Can you work these out from the model? Positions are in its coordinate system, mm. A direction names the side the tool comes from. Give positions to 0.01 mm unless a question says otherwise; leave off trailing zeros. Order: outer loops, then holes, each group sorted by start corner. A loop starts at its lowest first (then second) coordinate and runs counter-clockwise, first axis right, second up. Notation, with made-up numbers: (50, 11) - (105, 11) arc R19 cw to (105, 29) - close; hole circle Ø4 at (25, 64.25). An arc over 180 degrees is marked (long way). Answer as CSV lines item,"result".
```python
from build123d import *

# Parameters (mm, degrees)
SKETCH_1_R               = 2.5
EXTRUDE_1_DEPTH          = 4
EXTRUDE_2_DEPTH          = 15
SKETCH_3_W               = 28
SKETCH_3_H               = 4
CUT_EXTRUDE_1_DEPTH      = 8
CUT_EXTRUDE_2_DEPTH      = 60.149678768
CUT_EXTRUDE_2_DEPTH_BACK = 60.149678768


with BuildPart() as part:
    # 草图1 → 凸台-拉伸1 (new body)
    with BuildSketch(Plane(origin=(0, 0, 0), x_dir=(1, 0, 0), z_dir=(0, 1, 0))):
        with BuildLine():
            Line((-27.928932188, -4.947284101), (27.928932188, -4.947284101))
            ThreePointArc((27.928932188, -4.947284101), (32.548329851, -8.03386694), (31.464466094, -13.482818007))
            Line((31.464466094, -13.482818007), (3.535533906, -41.411750195))
            ThreePointArc((3.535533906, -41.411750195), (0, -42.87621629), (-3.535533906, -41.411750195))
            Line((-3.535533906, -41.411750195), (-31.464466094, -13.482818007))
            ThreePointArc((-31.464466094, -13.482818007), (-32.548329851, -8.03386694), (-27.928932188, -4.947284101))
        make_face()
        with Locations(Location((-25, -9.947284101, 0), (0, 0, 270))):
            Circle(SKETCH_1_R, mode=Mode.SUBTRACT)
        with Locations(Location((25, -9.947284101, 0), (0, 0, 270))):
            Circle(SKETCH_1_R, mode=Mode.SUBTRACT)
        with Locations(Location((0, -34.947284101, 0), (0, 0, 270))):
            Circle(SKETCH_1_R, mode=Mode.SUBTRACT)
    extrude(amount=EXTRUDE_1_DEPTH)

    # 草图2 → 凸台-拉伸2 (add)
    with BuildSketch(Plane(origin=(0, 0, 4.947284101), x_dir=(-1, 0, 0), z_dir=(0, 0, -1))):
        Polygon((-20, 4), (-8.452994616, 24), (8.452994616, 24), (20, 4), align=None)
    extrude(amount=-EXTRUDE_2_DEPTH)

    # 草图3 → 切除-拉伸1 (cut)
    with BuildSketch(Plane(origin=(0, 0, 4.947284101), x_dir=(-1, 0, 0), z_dir=(0, 0, -1))):
        with Locations((0, 2)):
            Rectangle(SKETCH_3_W, SKETCH_3_H)
    extrude(amount=-CUT_EXTRUDE_1_DEPTH, mode=Mode.SUBTRACT)

    # 草图4 → 切除-拉伸2 (cut, two sides: drawn at the far end of the back side and taken through both)
    with BuildSketch(Plane(origin=(0, 0, 0), x_dir=(0, 0, -1), z_dir=(1, 0, 0)).offset(-CUT_EXTRUDE_2_DEPTH_BACK)):
        Polygon((-19.947284101, 24), (-7.947284101, 24), (-19.947284101, 4), align=None)
    extrude(amount=CUT_EXTRUDE_2_DEPTH + CUT_EXTRUDE_2_DEPTH_BACK, mode=Mode.SUBTRACT)


solid = part.part
```
1) I'm going to push flat-ended pins straight in: P1, Ø8, axis at x = 11, y = 20, coming from the -Z side; P2, Ø1.2, axis at x = -2.5, y = 3, coming from the -Z side; P3, Ø3, axis at y = 2, z = 7.5, coming from the +X side; P4, Ø4, axis at x = 13.5, y = 3, coming from the +Z side. Where does each tip first touch, or does it pass through?
Answer block:
P1,"z = 4.95"
P2,"z = 12.95"
P3,"x = 32.84"
P4,"z = 33.45"
2) I need wall thicknesses on line 1 along Y through (x, z) = (14, 21.5); line 2 along X through (y, z) = (12.5, 7); line 3 along Y through (x, z) = (-6, 19). Which ranges of each line are inside material? Lowest first, please. Write a range as [from, to].
Answer block:
line 1,"[0, 4]"
line 2,"[-15.09, 15.09]"
line 3,"[0, 5.58]"
3) I want a section at B-B on y = 2.5. Write out the boundary of the cut face in (x, z), plus the area to 3 significant figures.
Answer block:
outline,"(-31.46, 13.48) arc R5 ccw to (-27.93, 4.95) - (-14, 4.95) - (-14, 12.95) - (14, 12.95) - (14, 4.95) - (27.93, 4.95) arc R5 ccw to (31.46, 13.48) - (3.54, 41.41) arc R5 ccw to (-3.54, 41.41) - close; hole circle Ø5 at (-25, 9.95); hole circle Ø5 at (0, 34.95); hole circle Ø5 at (25, 9.95)"
area,"1,250 mm2"
4) I want a section at D-D on x = 7. Write out the boundary of the cut face in (y, z).
Answer block:
outline,"(0, 12.95) - (4, 12.95) - (4, 4.95) - (24, 4.95) - (24, 7.95) - (4, 19.95) - (4, 37.95) - (0, 37.95) - close"
5) If we mould it in two halves opening along X, with no side actions, what happens to faces 4 (the flat face through (0, 2, 12.947)), 5 (the flat face through (15.59, 11.64, 10.68)), 6 (the cylindrical face through (-32.58, 1.97, 8.11))? For each: +X half, -X half, draft (parallel to the pull), parting line (faces both ways), or undercut.
Answer block:
face 4,"undercut"
face 5,"+X half"
face 6,"-X half"
6) I want a section at A-A on x = 0. Write out the boundary of the cut face in (y, z).
Answer block:
outline,"(0, 12.95) - (4, 12.95) - (4, 4.95) - (24, 4.95) - (24, 7.95) - (4, 19.95) - (4, 32.45) - (0, 32.45) - close; (0, 37.45) - (4, 37.45) - (4, 42.88) - (0, 42.88) - close"
7) Which directions (+Z, -Z, +X, -X, +Y, -Y) give clear straight access to the entire face, cutting with the end or side of a thin tool? Please do faces 1 (the flat face through (0, 4, 24)), 2 (the flat face through (-14, 2, 9)), 3 (the flat face through (0, 12, 4.947)).
Answer block:
face 1,"+Z, +Y"
face 2,"-Z, -Y"
face 3,"-Z, +X, -X, +Y, -Y"
8) I want a section at C-C on x = -25. Write out the boundary of the cut face in (y, z), plus the area to 3 significant figures.
Answer block:
outline,"(0, 4.95) - (4, 4.95) - (4, 7.45) - (0, 7.45) - close; (0, 12.45) - (4, 12.45) - (4, 19.95) - (0, 19.95) - close"
area,"40.0 mm2"
